from build123d import *

# Parameters (mm, degrees)
ESBO_O1_W                = 300
ESBO_O1_H                = 180
ESBO_O1_R                = 2
ESBO_O1_R_2              = 4
RESSALTO_EXTRUS_O1_DEPTH = 6
ESBO_O2_R                = 2
CORTE_EXTRUS_O1_DEPTH    = 10


with BuildPart() as part:
    # Esboço1 → Ressalto-extrusão1 (new body)
    with BuildSketch(Plane.XY):
        Rectangle(ESBO_O1_W, ESBO_O1_H)
        with Locations((120, -80)):
            Circle(ESBO_O1_R, mode=Mode.SUBTRACT)
        with Locations((140, 80)):
            Circle(ESBO_O1_R, mode=Mode.SUBTRACT)
        with Locations((-140, 80)):
            Circle(ESBO_O1_R, mode=Mode.SUBTRACT)
        with Locations((-140, -80)):
            Circle(ESBO_O1_R, mode=Mode.SUBTRACT)
        with Locations((-115, -64)):
            Circle(ESBO_O1_R_2, mode=Mode.SUBTRACT)
        with Locations((-35, -64)):
            Circle(ESBO_O1_R_2, mode=Mode.SUBTRACT)
    extrude(amount=RESSALTO_EXTRUS_O1_DEPTH)

    # Esboço2 → Corte-extrusão1 (cut)
    with BuildSketch(Plane.XY.offset(6)):
        with Locations((120, 72)):
            Circle(ESBO_O2_R)
        with Locations((-5.6, 72)):
            Circle(ESBO_O2_R)
        with Locations((-5.6, -13)):
            Circle(ESBO_O2_R)
        with Locations((120, -13)):
            Circle(ESBO_O2_R)
    extrude(amount=-CORTE_EXTRUS_O1_DEPTH, mode=Mode.SUBTRACT)


solid = part.part
Here's how the part is built. I have some questions about the finished solid (model axes, mm). Round coordinates to 2 decimals unless told otherwise and drop trailing zeros. Order: outer loops, then holes, each group sorted by start corner. A loop starts at its lowest first (then second) coordinate and runs counter-clockwise, first axis right, second up. Notation, with made-up numbers: M 23.25,8.25 L 75.25,8.25 A6 ccw 75.25,12.25 Z; hole C 60.5,63 d5. An arc over 180 degrees is marked long. Return JSON: item names as keys, results as strings. Group by question number.
1. I'm going to push a flat-ended pin straight in: pin 1 Ø6.5 at (x, y) = (-115, -64) entering from -Z. Where does the tip first touch, or does it pass through?
2. If we section it at B-B on x = -115: List the corners of the cut face in (y, z) for me, then the cut area to 3 significant figures.
3. If we mould it in two halves opening along Y, with no side actions, what happens to faces 1 (the face through (-35.867, -67.905, 2.958)), 2 (the face through (-2, 1, 6)), 3 (the face through (-2, 90, 3))? For each: pulls with the +Y half, pulls with the -Y half, needs draft (parallel to the pull), parting line crosses it, or undercut.
4. Please list where these lines run through material, in increasing order: probe 1 along Y at (x, z) = (-140, 2.85); probe 2 along Y at (x, z) = (120, 1.5); probe 3 along Y at (x, z) = (-35, 2.3).
5. If we section it at A-A on y = -64: List the corners of the cut face in (x, z) for me.
Reply:
{
 "1": {"pin 1": "through"},
 "2": {"outline": "M -90,0 L -68,0 L -68,6 L -90,6 Z; M -60,0 L 90,0 L 90,6 L -60,6 Z", "area": "1,030 mm^2"},
 "3": {"face 1": "undercut", "face 2": "needs draft", "face 3": "pulls with the +Y half"},
 "4": {"probe 1": "-90 to -82, -78 to 78, 82 to 90", "probe 2": "-90 to -82, -78 to -15, -11 to 70, 74 to 90", "probe 3": "-90 to -68, -60 to 90"},
 "5": {"outline": "M -150,0 L -119,0 L -119,6 L -150,6 Z; M -111,0 L -39,0 L -39,6 L -111,6 Z; M -31,0 L 150,0 L 150,6 L -31,6 Z"}
}
